Check sheet for the modelled part. Datum: model origin and axes. Units: mm. Face numbers are marked on the shaded views. A direction names the side the tool comes from. Round coordinates to 2 decimals unless told otherwise and drop trailing zeros. Write each loop counter-clockwise with the first axis right and the second up, starting at its lowest first coordinate (ties: lowest second). Pieces come first, ordered by that corner, then holes. Notation, with made-up numbers: (-22.75, 72) -> (14.25, 72) arc R26 cw to (14.25, 86) -> close; hole circle Ø11 at (18, 12.25). An arc over 180 degrees is marked (long way). Use one line per item in the form item = value. Start each with the question number.
```python
from build123d import *

# Parameters (mm, degrees)
SKETCH1_W           = 2.272369049
SKETCH1_H           = 2.138700281
BOSS_EXTRUDE1_DEPTH = 2.25
FILLET1_R           = 1


with BuildPart() as part:
    # Sketch1 → Boss-Extrude1 (new body)
    with BuildSketch(Plane(origin=(0, 0, 0), x_dir=(1, 0, 0), z_dir=(0, 1, 0))):
        Polygon((-17.128579952, 1.837543865), (-6.128579952, 21.087543865), (4.871420048, 1.837543865), align=None)
        Polygon((-7.264764476, 7.408947213), (-4.992395427, 7.408947213), (-4.463947201, 14.949533453), (-7.793212702, 14.949533453), align=None, mode=Mode.SUBTRACT)
        with Locations((-6.128579952, 4.848079389)):
            Rectangle(SKETCH1_W, SKETCH1_H, mode=Mode.SUBTRACT)
    extrude(amount=BOSS_EXTRUDE1_DEPTH)

    # Fillet1
    fillet1_edges = [part.edges().sort_by_distance(p)[0] for p in [
        (-17.128579952, 1.125, -1.837543865),
        (-6.128579952, 1.125, -21.087543865),
        (4.871420048, 1.125, -1.837543865),
    ]]
    fillet(fillet1_edges, radius=FILLET1_R)


solid = part.part
```
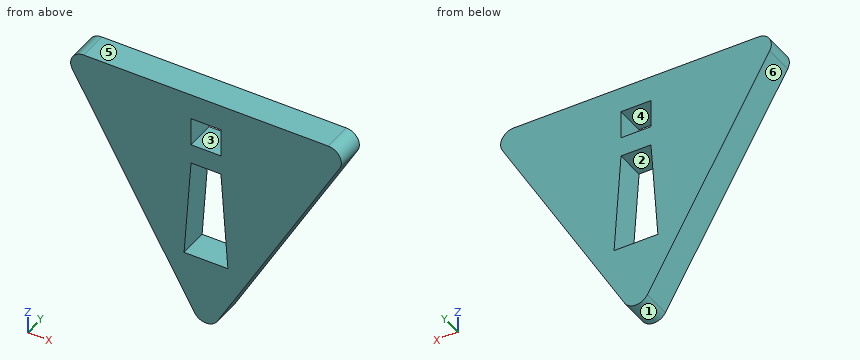
1. Sectioned sample at C-C (z = -5.5). Enter the section's corners in (x, y), and give its area (3 significant figures).
2. Sectioned sample at D-D (x = -10.5). Enter the section's corners in (y, z), and give its area (3 significant figures).
3. Sectioned sample at B-B (z = -10). Enter the section's corners in (x, y).
4. Mould release check, pull along Z, two halves, no side actions. Record for the marked faces 3, 4, 5 and 6: +Z half, -Z half, draft (parallel to the pull), parting line (faces both ways), or undercut.
5. Sectioned sample at A-A (y = 1.1). Enter the section's corners in (x, z).
6. Scan lines: probe 1 along Z at (x, y) = (-7, 0.8); probe 2 along Z at (x, y) = (-5.75, 0.25); probe 3 along X at (y, z) = (0.75, -5.5). Record each from-to range of solid material in increasing order.
7. Depth check by flat-ended pin: pin 1 (0.6 mm diameter, centred on y = 0.5, z = -5, fed in from -X); pin 2 (0.6 mm diameter, centred on y = 1, z = -5, fed in from +X). Enter the tip coordinate at first touch or a pass-through.
8. Tool access check on the marked faces 1 and 2. Record the directions out of +Z, -Z, +X, -X, +Y, -Y that give a thin tool (end or side, any length) a straight path to the whole face; none if there is none.
Returned:
q1.outline = (-15.04, 0) -> (-7.26, 0) -> (-7.26, 2.25) -> (-15.04, 2.25) -> close; (-4.99, 0) -> (2.78, 0) -> (2.78, 2.25) -> (-4.99, 2.25) -> close
q1.area = 35.0 mm^2
q2.outline = (0, -13.44) -> (2.25, -13.44) -> (2.25, -1.84) -> (0, -1.84) -> close
q2.area = 26.1 mm^2
q3.outline = (-12.46, 0) -> (-7.45, 0) -> (-7.45, 2.25) -> (-12.46, 2.25) -> close; (-4.81, 0) -> (0.21, 0) -> (0.21, 2.25) -> (-4.81, 2.25) -> close
q4.face_3 = undercut
q4.face_4 = undercut
q4.face_5 = +Z half
q4.face_6 = -Z half
q5.outline = (-16.27, -3.33) -> (-7, -19.57) arc R1 ccw to (-5.26, -19.57) -> (4.02, -3.33) arc R1 ccw to (3.15, -1.84) -> (-15.41, -1.84) arc R1 ccw to start; hole (-7.79, -14.95) -> (-4.46, -14.95) -> (-4.99, -7.41) -> (-7.26, -7.41) -> close; hole (-7.26, -5.92) -> (-4.99, -5.92) -> (-4.99, -3.78) -> (-7.26, -3.78) -> close
q6.probe_1 = -19.56 to -14.95, -7.41 to -5.92, -3.78 to -1.84
q6.probe_2 = -20 to -14.95, -7.41 to -5.92, -3.78 to -1.84
q6.probe_3 = -15.04 to -7.26, -4.99 to 2.78
q7.pin_1 = -15.49
q7.pin_2 = 3.24
q8.face_1 = -Z, +Y, -Y
q8.face_2 = +Y, -Y
